Autodesk Inventor part; units mm, degrees
ref_plane "YZ Plane" through (0, 0, 0) normal (1, 0, 0) x (0, 1, 0)
ref_plane "XZ Plane" through (0, 0, 0) normal (0, 1, 0) x (-1, 0, 0)
ref_plane "XY Plane" through (0, 0, 0) normal (0, 0, 1) x (1, 0, 0)
sketch "Sketch1" plane through (0, 0, 0) normal (0, 1, 0) x (-1, 0, 0)
  circle A0 centre (2.2, 0) radius 9.525
  circle A1 centre (-15.7605, -17.9605) radius 2.0193 construction
  circle A2 centre (20.1605, -17.9605) radius 2.0193 construction
  circle A3 centre (20.1605, 17.9605) radius 2.0193 construction
  circle A4 centre (-15.7605, 17.9605) radius 2.0193 construction
  circle A5 centre (2.2, -29.26) radius 15.5575 construction
  circle A6 centre (2.2, 29.26) radius 15.5575 construction
  circle A7 centre (-71, 10) radius 3 construction
  circle A8 centre (-71, -10) radius 3 construction
  line L0 (-93.1199, -15.5417) -> (-49.1294, -16.4557) construction
  line L1 (-49.1294, -16.4557) -> (-48.8801, -4.4583) construction
  line L2 (-92.8706, -3.5443) -> (-48.8801, -4.4583) construction
  line L3 (-93.1199, -15.5417) -> (-92.8706, -3.5443) construction
  line L4 (-25, 210) -> (-25, -210) construction
  line L5 (25, 210) -> (25, -210) construction
  arc A9 (17.6544, -25.1175) -> (-13.2881, -25.2451) centre (2.2, -29.26) ccw
  circle A10 centre (-71, -10) radius 9 construction
  circle A11 centre (-71, 10) radius 9 construction
  line L6 (23, -35) -> (-24.672, -35) construction
  line L7 (-24.672, 35) -> (23, 35) construction
  line L8 (25, -18.7054) -> (25, 18.7057)
  arc A12 (17.6544, -25.1175) -> (25, -18.7054) centre (2.2, 0) ccw
  arc A13 (-13.2544, -25.1175) -> (-12.7349, -35) centre (2.2, -29.26) ccw
  arc A14 (-12.7349, 35) -> (17.6545, 25.1177) centre (2.2, 29.26) ccw
  arc A15 (25, 18.7057) -> (17.6545, 25.1177) centre (2.2, 0) ccw
  line L9 (-12.7349, -35) -> (-24.672, -35)
  line L10 (-12.7349, 35) -> (-24.672, 35)
  line L11 (-24.672, -35) -> (-73.8571, -18.5345)
  line L12 (-24.672, 35) -> (-73.8571, 18.5345)
  line L13 (-80, -10) -> (-80, 10)
  arc A16 (-80, -10) -> (-73.8571, -18.5345) centre (-71, -10) ccw
  arc A17 (-73.8571, 18.5345) -> (-80, 10) centre (-71, 10) ccw
  line L14 (-58.5968, -11.0143) -> (-31.5968, -20.1136)
  arc A18 (-62, -6.2761) -> (-58.5968, -11.0143) centre (-57, -6.2761) ccw
  line L15 (-62, 6.2761) -> (-62, -6.2761)
  arc A19 (-58.5968, 11.0143) -> (-62, 6.2761) centre (-57, 6.2761) ccw
  line L16 (-31.5968, 20.1136) -> (-58.5968, 11.0143)
  arc A20 (-25, 15.3755) -> (-31.5968, 20.1136) centre (-30, 15.3755) ccw
  arc A21 (-31.5968, -20.1136) -> (-25, -15.3755) centre (-30, -15.3755) ccw
  arc A22 (-25, 11.397) -> (-25, -11.397) centre (2.2, 0) ccw
  line L17 (-25, -15.3755) -> (-25, -11.397)
  line L18 (-25, 15.3755) -> (-25, 11.397)
  arc A23 (-18.6534, -20.8534) -> (23.0534, 20.8534) centre (2.2, 0) ccw
  spline S0 degree 3 poles (23.0534, 20.8534) (21.798, 22.1089) (20.4403, 23.2417) (18.9803, 24.2518) (18.9572, 24.2679) (18.9354, 24.2829) (18.9107, 24.2998) (17.3595, 25.3666) (15.7211, 26.2765) (13.9955, 27.0296) (13.9681, 27.0415) (13.9418, 27.0529) (13.9132, 27.0653) (12.1415, 27.8321) (10.3123, 28.4192) (8.4258, 28.8266) (8.3649, 28.8397) (8.3053, 28.8524) (8.243, 28.8654) (6.2506, 29.2826) (4.2356, 29.4912) (2.2, 29.4912) (0.228, 29.4912) (-1.724, 29.2955) (-3.6561, 28.9039) (-3.7184, 28.8913) (-3.7821, 28.8782) (-3.843, 28.8654) (-5.7631, 28.4635) (-7.6246, 27.8758) (-9.4274, 27.1023) (-9.456, 27.09) (-9.4858, 27.0772) (-9.5132, 27.0653) (-11.241, 26.3176) (-12.8822, 25.4127) (-14.4368, 24.3505) (-14.4614, 24.3337) (-14.4875, 24.3158) (-14.5107, 24.2998) (-15.9968, 23.278) (-17.3782, 22.1287) (-18.6534, 20.8534) (-19.9088, 19.5981) (-21.0416, 18.2404) (-22.0518, 16.7803) (-22.0679, 16.7572) (-22.0829, 16.7354) (-22.0998, 16.7107) (-23.1666, 15.1595) (-24.0765, 13.5211) (-24.8296, 11.7955) (-24.8415, 11.7681) (-24.8529, 11.7418) (-24.8653, 11.7132) (-25.6321, 9.9415) (-26.2192, 8.1123) (-26.6266, 6.2258) (-26.6397, 6.1649) (-26.6524, 6.1053) (-26.6654, 6.043) (-27.0826, 4.0506) (-27.2912, 2.0356) (-27.2912, 0) (-27.2912, -1.972) (-27.0955, -3.924) (-26.7039, -5.8561) (-26.6913, -5.9184) (-26.6782, -5.9821) (-26.6654, -6.043) (-26.2635, -7.9631) (-25.6758, -9.8246) (-24.9023, -11.6274) (-24.89, -11.656) (-24.8772, -11.6858) (-24.8653, -11.7132) (-24.1176, -13.441) (-23.2127, -15.0822) (-22.1505, -16.6368) (-22.1337, -16.6614) (-22.1158, -16.6875) (-22.0998, -16.7107) (-21.0779, -18.1969) (-19.929, -19.5778) (-18.6534, -20.8534) knots 0 0 0 0 0.061523 0.061523 0.061523 0.0625 0.0625 0.0625 0.124023 0.124023 0.124023 0.125 0.125 0.125 0.185547 0.185547 0.185547 0.1875 0.1875 0.1875 0.25 0.25 0.25 0.310547 0.310547 0.310547 0.3125 0.3125 0.3125 0.374023 0.374023 0.374023 0.375 0.375 0.375 0.436523 0.436523 0.436523 0.4375 0.4375 0.4375 0.5 0.5 0.5 0.561523 0.561523 0.561523 0.5625 0.5625 0.5625 0.624023 0.624023 0.624023 0.625 0.625 0.625 0.685547 0.685547 0.685547 0.6875 0.6875 0.6875 0.75 0.75 0.75 0.810547 0.810547 0.810547 0.8125 0.8125 0.8125 0.874023 0.874023 0.874023 0.875 0.875 0.875 0.936523 0.936523 0.936523 0.9375 0.9375 0.9375 1 1 1 1
  point P0 (0, 0)
  point P1 (-13.2881, -25.2451)
  dimension "d4" = 16
  dimension "d5" = 18
  dimension "d6" = 18
  dimension "d7" = 16
extrude "Extrusion1" add sketch "Sketch1" against normal blind 5 contours A9 A23 S0 A22 A14 A15 L8 A12 | A9 A13 L9 L11 A16 L13 A17 L12 L10 A14 S0 L18 A20 L16 A19 L15 A18 L14 A21 L17 A23
fillet "Fillet1" radius 5 2 edges at (25, -2.5, 11.397) (25, -2.5, -11.397)
fillet "Fillet2" radius 2 8 edges at (12.7349, -2.5, 35) (-17.6545, -2.5, 25.1177) (-17.6544, -2.5, -25.1175) (12.7349, -2.5, -35) (24.672, -2.5, -35) (24.672, -2.5, 35) (-25, -2.5, -18.7054) (-25, -2.5, 18.7057)
sketch "Sketch2" plane through (0, 0, 0) normal (0, 1, 0) x (1, 0, 0)
  circle A0 centre (71, 10) radius 3
  circle A1 centre (71, -10) radius 3
  point P0 (0, 0)
hole "Hole1" at (71, 0, -10) at (71, 0, 10) direction (0, -1, 0) diameter 6 end through all
sketch "Sketch3" plane through (0, 0, 0) normal (0, 1, 0) x (1, 0, 0)
  point P0 (0, 0)
sketch "Sketch4" plane through (0, 0, 0) normal (0, 1, 0) x (1, 0, 0)
  circle A0 centre (-20.1605, -17.9605) radius 3
  circle A1 centre (15.7605, 17.9605) radius 3
  circle A2 centre (15.7605, -17.9605) radius 3
  circle A3 centre (-20.1605, 17.9605) radius 3
  circle A4 centre (-4, -61.01) radius 14.2875
  circle A5 centre (-2.2, 29.26) radius 14.2875
  circle A6 centre (-2.2, -29.26) radius 14.2875
  circle A7 centre (-4, 61.01) radius 14.2875
  circle A8 centre (-2.2, 0) radius 9.5
  line L0 (-25, -210) -> (25, -210)
  line L1 (25, -210) -> (25, 210)
  line L2 (-25, 210) -> (25, 210)
  line L3 (-25, -210) -> (-25, 210)
  point P0 (0, 0)
hole "Hole2" at (15.7605, 0, -17.9605) at (15.7605, 0, 17.9605) at (-20.1605, 0, 17.9605) at (-20.1605, 0, -17.9605) direction (0, -1, 0) diameter 5 depth 8 tip angle 118
properties part number "pistonplatefront"
Could you check a few things on this model? Use its own coordinates, in mm. A direction names the side the tool comes from. Coordinates: 2 decimals unless noted, no trailing zeros. Loops run counter-clockwise (first coordinate to the right, second up) from the corner with the lowest first, then second, coordinate; pieces in that order, holes last.
1. We'd pull the mould along X, two halves only. Please class faces 1 (the face through (49.08, -2.46, 26.83)), 2 (the face through (44.908, -2.465, 15.628)), 3 (the face through (-22.28, -2.46, -21.6)): released by +X, released by -X, zero draft, split by the parting line, or undercut.
2. Imagine slicing it at C-C (z = -21.5). Please give me the cut outline in (x, y), and give its area (3 significant figures).
3. For faces 4 (the face through (27.137, -2.465, -19.475)), 5 (the face through (20, -2, -35)), which set-ups out of +Z, -Z, +X, -X, +Y, -Y let a thin tool reach every point of the face, with its end or its side?
4. Imagine slicing it at A-A (x = -2.2). Please give me the cut outline in (y, z) (3 decimals), and give its area (3 significant figures).
5. Imagine slicing it at D-D (x = 64.5). Please give me the cut outline in (y, z).
6. For P1, Ø8, axis at x = 15.76, z = 17.96, coming from the -Y side; P2, Ø1.5, axis at x = 9.5, y = -3.5, coming from the -Z side; P3, Ø1, axis at x = 53.5, y = -1.5, coming from the +Z side, each with a flat end and sliding along its axis, tell me the tip position at first contact or that it passes through.
7. Imagine slicing it at B-B (z = 0). Please give me the cut outline in (x, y) (3 decimals), and give its area (3 significant figures).
8. I need wall thicknesses on L1, parallel to Z at x = -19, y = -3.3; L2, parallel to X at y = -4.7, z = 0.5; L3, parallel to Z at x = 71, y = -1.8. Which ranges of each line are inside material? Lowest first, please.
Computed values:
1. face 1: released by +X
1. face 2: undercut
1. face 3: released by -X
2. outline: (-22.39, -5) - (-16.19, -5) - (-16.19, 0) - (-22.39, 0) - close; (11.79, -5) - (65, -5) - (65, 0) - (11.79, 0) - close
2. area: 297 mm2
3. face 4: +Y, -Y
3. face 5: -Z, +X, -X, +Y, -Y
4. outline: (-5, -13.26) - (0, -13.26) - (0, -9.525) - (-5, -9.525) - close; (-5, 9.525) - (0, 9.525) - (0, 13.26) - (-5, 13.26) - close
4. area: 37.4 mm2
5. outline: (-5, -21.67) - (0, -21.67) - (0, 21.67) - (-5, 21.67) - close
6. P1: stops at y = -5
6. P2: stops at z = -19.21
6. P3: stops at z = 25.52
7. outline: (-25, -5) - (-11.725, -5) - (-11.725, 0) - (-25, 0) - close; (7.325, -5) - (27.291, -5) - (27.291, 0) - (7.325, 0) - close; (62, -5) - (80, -5) - (80, 0) - (62, 0) - close
7. area: 256 mm2
8. L1: z = -23.98 to -20.17, -15.75 to 15.75, 20.17 to 23.98
8. L2: x = -25 to -11.71, 7.31 to 27.29, 62 to 80
8. L3: z = -19.49 to -13, -7 to 7, 13 to 19.49
